Drawing for the job (mm, zero at the part's lowest x, y, z). Give positions to 0.01 mm unless a question says otherwise; leave off trailing zeros. Write each loop counter-clockwise with the first axis right and the second up, starting at its lowest first coordinate (ties: lowest second). Pieces come first, ordered by that corner, then holes. Notation, with made-up numbers: M 37.5,-24 L 53.5,-24 A20 ccw 53.5,2 Z; hole C -36.75,68.5 d2. An arc over 180 degrees is marked long. Use a Markdown table: item, result. Add a question column.
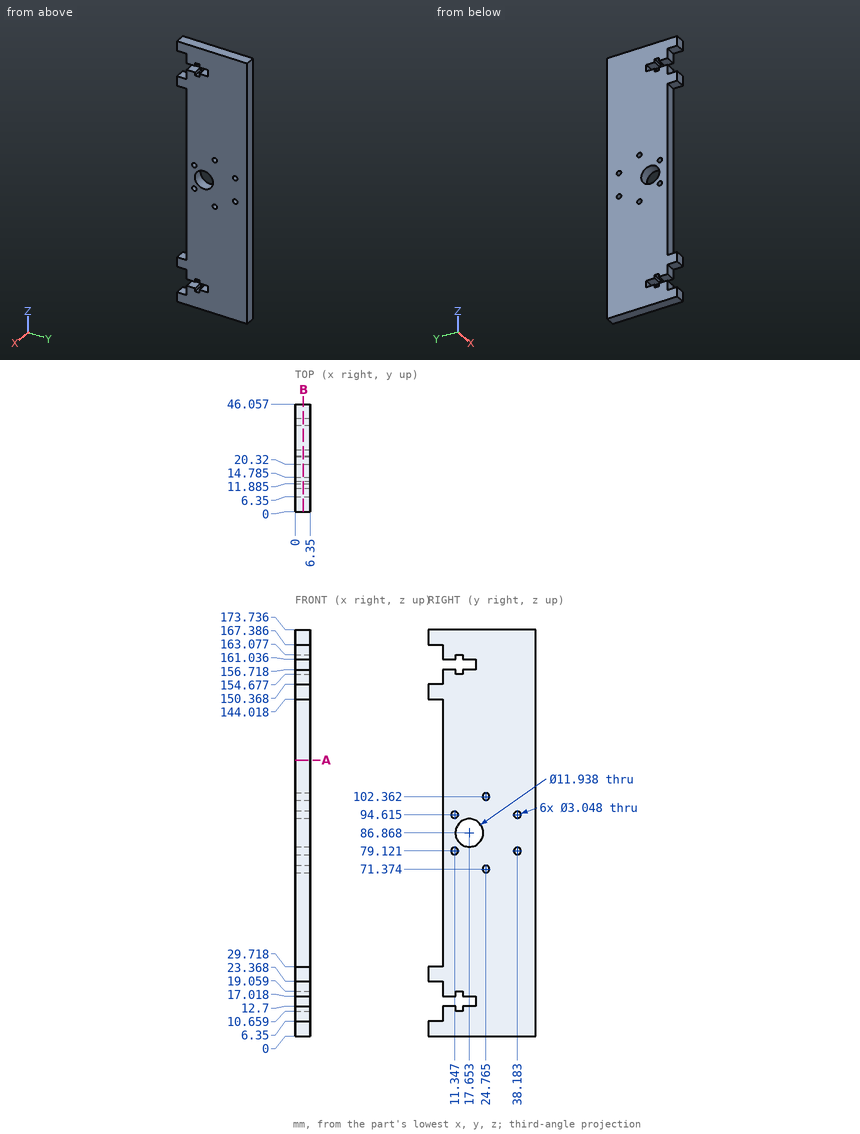
1. Cut at A-A (z = 118). Write the cut outline in (x, y), then the cut area to 3 significant figures.
2. Drill centre lines: probe 1 along Z at (x, y) = (1.75, 4); probe 2 along Z at (x, y) = (5.25, 25); probe 3 along Z at (x, y) = (3.5, 14) (1 decimal). Where is each one in solid material? Low to high. Write a range as [from, to].
3. Cut at B-B (x = 3.5). Give the number of separate pieces and of enclosed holes in the cut face, then the cut area to 3 significant figures.
4. Flat gauge pin, fed straight in: pin 1 (2 mm diameter, centred on x = 4.5, z = 156, fed in from -Y). Where does the tip first touch, or does it go through?
A:
| question | item | result |
|---|---|---|
| 1 | outline | M 0,6.35 L 6.35,6.35 L 6.35,46.06 L 0,46.06 Z |
| 1 | area | 252 mm² |
| 2 | probe 1 | z = [0, 6.35], [23.37, 29.72], [144.02, 150.37], [167.39, 173.74] |
| 2 | probe 2 | z = [0, 69.87], [72.88, 100.86], [103.87, 173.74] |
| 2 | probe 3 | z = [0, 10.7], [19.1, 82.1], [91.6, 154.7], [163.1, 173.7] |
| 3 | separate pieces | 1 |
| 3 | enclosed holes | 7 |
| 3 | area | 6,760 mm² |
| 4 | pin 1 | stops at y = 6.35 |
